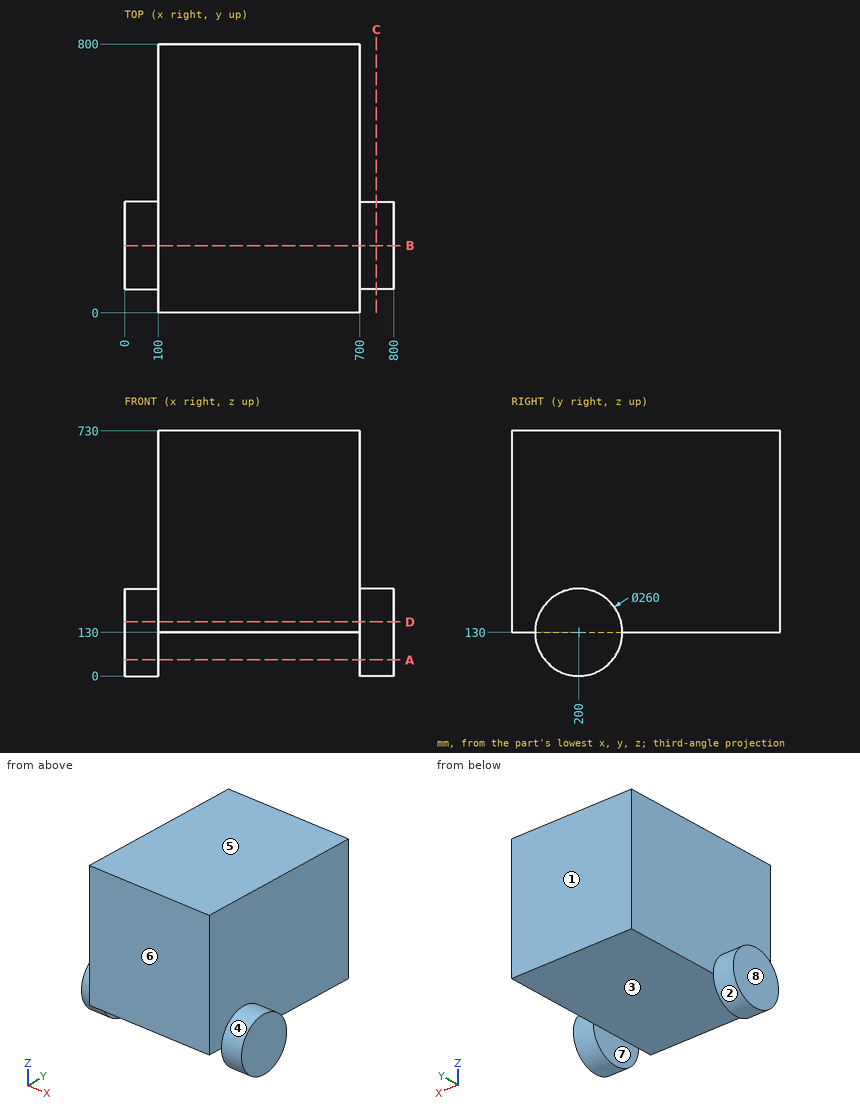
Verification items for this drawing (mm, ordinates from the low corner). A direction names the side the tool comes from. Round coordinates to 2 decimals unless told otherwise and drop trailing zeros. Write each loop counter-clockwise with the first axis right and the second up, starting at its lowest first coordinate (ties: lowest second). Pieces come first, ordered by that corner, then holes. Notation, with made-up numbers: M -3.5,-4.75 L 1.5,-4.75 A9 ccw 1.5,0.25 Z; hole C -17,-14 d10. An arc over 180 degrees is marked long. Write item = value, one per line. Start each with the question number.
1. Scan lines: line 1 (X direction, y = 55.5, z = 205); line 2 (Z direction, x = 574, y = 392); line 3 (Z direction, x = 732.5, y = 235). Record each from-to range of solid material in increasing order. Write a range as [from, to].
2. Section check C-C, the plane x = 749. Record the cut outline in (y, z), then the cut area to 3 significant figures.
3. Tool access check on the marked faces 1, 2, 3, 4 and 5. Record the directions out of +Z, -Z, +X, -X, +Y, -Y that give a thin tool (end or side, any length) a straight path to the whole face; none if there is none.
4. Release check for a two-part mould opening along X. For the marked faces 6, 7 and 8 record: pulls with the +X half, pulls with the -X half, needs draft (parallel to the pull), parting line crosses it, or undercut.
5. Gauge pin test, flat ends, axial feed: pin 1 (10 mm diameter, centred on y = 366.5, z = 167, fed in from +X); pin 2 (12 mm diameter, centred on x = 544.5, y = 382, fed in from -Z); pin 3 (1 mm diameter, centred on x = 700, y = 109, fed in from -Z). Record the tip position at first contact, or that the pin passes through.
6. Section check D-D, the plane z = 161. Record the cut outline in (x, y).
7. Section check A-A, the plane z = 48. Record the cut outline in (x, y), then the cut area to 3 significant figures.
8. Section check B-B, the plane y = 200. Record the cut outline in (x, z).
Results found:
q1.line_1 = [100, 700]
q1.line_2 = [130, 730]
q1.line_3 = [4.8, 255.2]
q2.outline = C 200,130 d260
q2.area = 53,100 mm^2
q3.face_1 = +Z, -Z, +X, -X, +Y
q3.face_2 = -X
q3.face_3 = -Z, +Y, -Y
q3.face_4 = +X
q3.face_5 = +Z, +X, -X, +Y, -Y
q4.face_6 = needs draft
q4.face_7 = undercut
q4.face_8 = pulls with the -X half
q5.pin_1 = 700
q5.pin_2 = 130
q5.pin_3 = 36.67
q6.outline = M 0,73.75 L 100,73.75 L 100,0 L 700,0 L 700,73.75 L 800,73.75 L 800,326.25 L 700,326.25 L 700,800 L 100,800 L 100,326.25 L 0,326.25 Z
q7.outline = M 0,99.12 L 100,99.12 L 100,300.88 L 0,300.88 Z; M 700,99.12 L 800,99.12 L 800,300.88 L 700,300.88 Z
q7.area = 40,400 mm^2
q8.outline = M 0,0 L 100,0 L 100,130 L 700,130 L 700,0 L 800,0 L 800,260 L 700,260 L 700,730 L 100,730 L 100,260 L 0,260 Z
